Source: CAD feature listing. Evaluate the final solid. Frame: model axes, mm. A direction names the side the tool comes from. Give positions to 0.01 mm unless a question says otherwise; leave off trailing zeros. Loops run counter-clockwise (first coordinate to the right, second up) from the corner with the lowest first, then second, coordinate; pieces in that order, holes last. Notation, with made-up numbers: M 72.25,49 L 94.25,49 A30 cw 94.25,86 Z; hole C 81,54.25 d9. An arc over 180 degrees is marked long. Answer in a Markdown table with one row per item.
```python
from build123d import *

# Parameters (mm, degrees)
F1_DEPTH = 25.4
F2_T     = -3.175


# Not quite as in the source:
# - ends of sketch curves that miss each other by under 0.0002 mm in the source are joined


with BuildPart() as f1:
    # F0 (on Front) → F1 (new body)
    with BuildSketch(Plane.XZ):
        with BuildLine():
            ThreePointArc((-46.9588833262, -52.3874997171), (0, -92.075), (46.9588833262, -52.3874997171))
            Line((46.9588833262, -52.3874997171), (59.4812628, 21.6958164))
            ThreePointArc((59.4812628, 21.6958164), (0, 92.075), (-59.4812496656, 21.6958186201))
            Line((-59.4812496656, 21.6958186201), (-46.9588833262, -52.3874997171))
        make_face()
    extrude(amount=F1_DEPTH)

    # F2
    f2_openings = [f1.faces().sort_by_distance(p)[0] for p in [
        (4e-06, -25.4, 3.213538),
    ]]
    offset(amount=F2_T, openings=f2_openings, kind=Kind.INTERSECTION)


solid = f1.part
```
Q1. Section query B-B (x = 25.5). Output: boundary loops of the cut face in (y, z) (3 decimals).
Values follow:
| item | result |
|---|---|
| outline | M -25.4,-84.673 L 0,-84.673 L 0,86.42 L -25.4,86.42 L -25.4,82.896 L -3.175,82.896 L -3.175,-80.858 L -25.4,-80.858 Z |
Q2. Ray query, probe 1 along Z at (x, y) = (-0.5, -7.75); probe 2 along Y at (x, z) = (36, 46) (3 decimals); probe 3 along Z at (x, y) = (8, -10.75). Return the intervals inside material, ascending. Write a range as from..to.
Values follow:
| item | result |
|---|---|
| probe 1 | -92.07..-88.9, 88.9..92.07 |
| probe 2 | -3.175..0 |
| probe 3 | -91.4..-88.17, 88.34..91.54 |
Q3. Contact query for flat-ended pins moving along their axis: pin 1 Ø4 at (x, z) = (10, 48.5) entering from -Y (3 decimals); pin 2 Ø3 at (x, y) = (-6.5, -8.5) entering from +Z; pin 3 Ø8 at (y, z) = (-10, -41.5) entering from -X. Output: stop coordinate, or through.
Values follow:
| item | result |
|---|---|
| pin 1 | y = -3.175 |
| pin 2 | z = 91.87 |
| pin 3 | x = -49.48 |
Q4. Reachability of faces 4 (the flat face through (-1, 0, 1)), 5 (the flat face through (-50.177, -14.132, -14.298)) from +Z, -Z, +X, -X, +Y, -Y: full face, straight path, thin tool, end or side. Return the list, or none.
Values follow:
| item | result |
|---|---|
| face 4 | +Z, -Z, +X, -X, +Y |
| face 5 | -Y |
Q5. Section query C-C (z = 14). Output: boundary loops of the cut face in (x, y) (3 decimals).
Values follow:
| item | result |
|---|---|
| outline | M -58.18,-25.4 L -54.96,-25.4 L -54.96,-3.175 L 54.96,-3.175 L 54.96,-25.4 L 58.18,-25.4 L 58.18,0 L -58.18,0 Z |
Q6. Mould query, pull axis Z, two halves, no side actions, for faces 1 (the flat face through (53, -25.4, 0)), 2 (the flat face through (50, -14.13, -15.34)), 3 (the cylindrical face through (-0.936, -12.522, -92.066)). Classes: +Z half, -Z half, draft (parallel to the pull), parting line (faces both ways), or undercut.
Values follow:
| item | result |
|---|---|
| face 1 | draft |
| face 2 | undercut |
| face 3 | -Z half |
